from build123d import *

# Parameters (mm, degrees)
SKETCH_1_R      = 1.5
EXTRUDE_1_DEPTH = 3


with BuildPart() as part:
    # Sketch 1 → Extrude 1 (new body)
    with BuildSketch(Plane(origin=(0, 0, 0), x_dir=(1, 0, 0), z_dir=(0, 1, 0))):
        with BuildLine():
            Line((61.023746461, 33.569203074), (61.021952874, 33.604841535))
            Line((61.021952874, 33.604841535), (58.025203482, 33.466081538))
            Line((58.025203482, 33.466081538), (57.840187699, 37.461800392))
            Line((57.840187699, 37.461800392), (73.823063114, 38.201863527))
            Line((73.823063114, 38.201863527), (74.008078898, 34.206144673))
            Line((74.008078898, 34.206144673), (71.011329506, 34.067384676))
            ThreePointArc((71.011329506, 34.067384676), (49.082411457, -9.842070835), (0.164945446, -13.841976975))
            ThreePointArc((0.164945446, -13.841976975), (-2.286053035, -7.209284728), (4.346639213, -4.758286247))
            ThreePointArc((4.346639213, -4.758286247), (43.480612021, -1.558361335), (61.023746461, 33.569203074))
        make_face()
        with Locations(Location((47.537682651, -4.519860589, 0), (0, 0, 270))):
            Circle(SKETCH_1_R, mode=Mode.SUBTRACT)
        with Locations(Location((19.224207172, -13.390815296, 0), (0, 0, 270))):
            Circle(SKETCH_1_R, mode=Mode.SUBTRACT)
    extrude(amount=EXTRUDE_1_DEPTH)


solid = part.part
Here's how the part is built. I have some questions about the finished solid (model axes, mm). A direction names the side the tool comes from. Coordinates: 2 decimals unless noted, no trailing zeros. Order: outer loops, then holes, each group sorted by start corner. A loop starts at its lowest first (then second) coordinate and runs counter-clockwise, first axis right, second up. Notation, with made-up numbers: M 24,44.25 L 63,44.25 A25 ccw 63,62.25 Z; hole C 4.25,-28.75 d11. An arc over 180 degrees is marked long. Answer as CSV lines item,"result".
Item 1: Imagine slicing it at C-C on x = 66.5. Write out the boundary of the cut face in (y, z), plus the area to 3 significant figures.
Results found:
outline,"M 0,-37.86 L 3,-37.86 L 3,-10.69 L 0,-10.69 Z"
area,"81.5 mm2"
Item 2: We'd pull the mould along Z, two halves only. Please class faces 1 (the face through (-2.33, 1.48, 7.31)), 2 (the face through (57.934, 1.479, -35.436)), 3 (the face through (47, 0, 0)), 4 (the face through (73.914, 1.479, -36.232)): +Z half, -Z half, draft (parallel to the pull), parting line (faces both ways), or undercut.
Results found:
face 1,"parting line"
face 2,"undercut"
face 3,"draft"
face 4,"-Z half"
Item 3: Imagine slicing it at B-B on z = -30. Write out the boundary of the cut face in (x, y), plus the area to 3 significant figures.
Results found:
outline,"M 61.04,0 L 71.05,0 L 71.05,3 L 61.04,3 Z"
area,"30.0 mm2"
Item 4: Imagine slicing it at A-A on y = 0.85. Give the number of separate pieces and of enclosed holes in the cut face, plus the area to 3 significant figures.
Results found:
separate pieces,"1"
enclosed holes,"2"
area,"1,010 mm2"
Item 5: For pin 1 (12 mm diameter, centred on x = 56, z = -20.5, fed in from -Y), with a flat end and sliding along its axis, tell me the tip position at first contact or that it passes through.
Results found:
pin 1,"y = 0"
Item 6: If I drill on line 1 (X direction, y = 2.3, z = 5.5); line 2 (X direction, y = 2.2, z = 5); line 3 (X direction, y = 2.6, z = -30.5), over which ranges is the centre line in solid material (lowest first)?
Results found:
line 1,"-0.99 to 6.06, 36.08 to 46.4, 48.67 to 54.62"
line 2,"-0.3 to 4.88, 37.26 to 46.12, 48.96 to 55.16"
line 3,"61.06 to 71.06"
Item 7: On a 3-axis mill with a long thin cutter (end or side, diameter ignored), from which of +Z, -Z, +X, -X, +Y, -Y can I reach the whole of each face in a straight line? I mean faces 5 (the face through (65.72, 1.479, -37.827)), 6 (the face through (43, 1.48, 1.88)). Say none if no direction works.
Results found:
face 5,"-Z, -X, +Y, -Y"
face 6,"+Y, -Y"
